from build123d import *

# Parameters (mm, degrees)
SKETCH1_W           = 30
SKETCH1_H           = 27.4
SKETCH1_R           = 5.15
BOSS_EXTRUDE1_DEPTH = 10
SKETCH2_R           = 2
CUT_EXTRUDE1_DEPTH  = 10
SKETCH7_R           = 1.2
CUT_EXTRUDE2_DEPTH  = 11


with BuildPart() as part:
    # Sketch1 → Boss-Extrude1 (new body)
    with BuildSketch(Plane.XY):
        with Locations((0, -2.7)):
            Rectangle(SKETCH1_W, SKETCH1_H)
        Circle(SKETCH1_R, mode=Mode.SUBTRACT)
    extrude(amount=BOSS_EXTRUDE1_DEPTH)

    # Sketch2 → Cut-Extrude1 (cut)
    with BuildSketch(Plane.XZ.offset(16.4)):
        with Locations((-11, 5)):
            Circle(SKETCH2_R)
        with Locations((11, 5)):
            Circle(SKETCH2_R)
    extrude(amount=-CUT_EXTRUDE1_DEPTH, mode=Mode.SUBTRACT)

    # Sketch7 → Cut-Extrude2 (cut, through all)
    with BuildSketch(Plane.XY.offset(10)):
        with Locations((-8, 0)):
            Circle(SKETCH7_R)
        with Locations((8, 0)):
            Circle(SKETCH7_R)
    extrude(amount=-CUT_EXTRUDE2_DEPTH, mode=Mode.SUBTRACT)


solid = part.part
Check sheet for the modelled part. Datum: model origin and axes. Units: mm. A direction names the side the tool comes from. Give positions to 0.01 mm unless a question says otherwise; leave off trailing zeros. Order: outer loops, then holes, each group sorted by start corner. A loop starts at its lowest first (then second) coordinate and runs counter-clockwise, first axis right, second up. Notation, with made-up numbers: M 65,-1 L 117,-1 A9 ccw 117,16 Z; hole C -32,-29 d10. An arc over 180 degrees is marked long. Answer as CSV lines item,"result". Start each with the question number.
Item 1: Cross-section at A-A on x = 0. Enter the section's corners in (y, z), plus the area to 3 significant figures.
Item 2: Mould release check, pull along X, two halves, no side actions. Record for faces 1 (the face through (11, -6.4, 5)), 2 (the face through (-15, -3, 5)), 3 (the face through (0, -6, 10)): +X half, -X half, draft (parallel to the pull), parting line (faces both ways), or undercut.
Item 3: Cross-section at C-C on z = 5. Enter the section's corners in (x, y), plus the area to 3 significant figures.
Item 4: Gauge pin test, flat end, axial feed: P1, Ø3, axis at x = -11, z = 5, coming from the -Y side. Record the tip position at first contact, or that the pin passes through.
Item 5: Cross-section at B-B on y = 0. Enter the section's corners in (x, z).
Item 6: Cross-section at D-D on x = -11. Enter the section's corners in (y, z).
Item 7: Tool access check on faces 4 (the face through (9, -11, 5)), 5 (the face through (-9.2, 0.05, 5.07)). Record the directions out of +Z, -Z, +X, -X, +Y, -Y that give a thin tool (end or side, any length) a straight path to the whole face; none if there is none.
Item 8: Thickness scan on line 1 (Y direction, x = 8, z = 7); line 2 (Z direction, x = -11, y = -6.75); line 3 (Y direction, x = 9, z = 2.75). Record the ranges inside material, lowest first. Write a range as [from, to].
Established:
1,outline,"M -16.4,0 L -5.15,0 L -5.15,10 L -16.4,10 Z; M 5.15,0 L 11,0 L 11,10 L 5.15,10 Z"
1,area,"171 mm^2"
2,face 1,"undercut"
2,face 2,"-X half"
2,face 3,"draft"
3,outline,"M -15,-16.4 L -13,-16.4 L -13,-6.4 L -9,-6.4 L -9,-16.4 L 9,-16.4 L 9,-6.4 L 13,-6.4 L 13,-16.4 L 15,-16.4 L 15,11 L -15,11 Z; hole C -8,0 d2.4; hole C 0,0 d10.3; hole C 8,0 d2.4"
3,area,"650 mm^2"
4,P1,"stops at y = -6.4"
5,outline,"M -15,0 L -9.2,0 L -9.2,10 L -15,10 Z; M -6.8,0 L -5.15,0 L -5.15,10 L -6.8,10 Z; M 5.15,0 L 6.8,0 L 6.8,10 L 5.15,10 Z; M 9.2,0 L 15,0 L 15,10 L 9.2,10 Z"
6,outline,"M -16.4,0 L 11,0 L 11,10 L -16.4,10 L -16.4,7 L -6.4,7 L -6.4,3 L -16.4,3 Z"
7,face 4,"-Y"
7,face 5,"+Z, -Z"
8,line 1,"y = [-16.4, -1.2], [1.2, 11]"
8,line 2,"z = [0, 3], [7, 10]"
8,line 3,"y = [-16.4, -0.66], [0.66, 11]"
